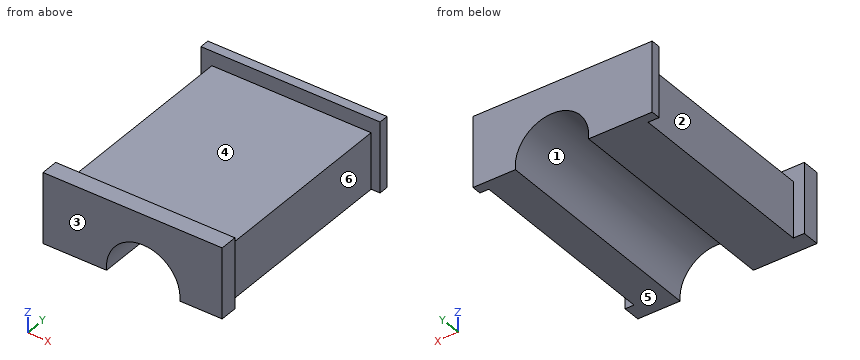
from build123d import *

# Parameters (mm, degrees)
F1_DEPTH = 80
F2_W     = 70.4753454775
F2_H     = 5.0733083159
F3_DEPTH = 64
F4_W     = 3.8940757513
F4_H     = 70.4753454775
F5_DEPTH = 25
F4_W_2   = 3.1526088715
F6_DEPTH = 25


with BuildPart() as f1:
    # F0 (on Front) → F1 (new body)
    with BuildSketch(Plane.XZ):
        with BuildLine():
            Line((-37.5057458878, 24.8617598087), (-37.5057458878, 0))
            Line((-37.5057458878, 0), (-15.074656345, 0))
            ThreePointArc((-15.074656345, 0), (-2.17074994, 14.2445032908), (10.733156465, 0))
            Line((10.733156465, 0), (25.6872158498, 0))
            Line((25.6872158498, 0), (25.6872158498, 24.8617598087))
            Line((25.6872158498, 24.8617598087), (-37.5057458878, 24.8617598087))
        make_face()
    extrude(amount=F1_DEPTH)

    # F2 (on face) → F3 (cut)
    with BuildSketch(Plane(origin=(-37.5057458878, 0, 0), x_dir=(0, -1, 0), z_dir=(-1, 0, 0))):
        with Locations((38.6002035812, 22.3251056507)):
            Rectangle(F2_W, F2_H)
    extrude(amount=-F3_DEPTH, mode=Mode.SUBTRACT)

    # F4 (on face) → F5 (cut)
    with BuildSketch(Plane.XY.offset(19.7884514928)):
        with Locations((-35.5587080121, -38.6002035812)):
            Rectangle(F4_W, F4_H)
    extrude(amount=-F5_DEPTH, mode=Mode.SUBTRACT)

    # F4 (on face) → F6 (cut)
    with BuildSketch(Plane.XY.offset(19.7884514928)):
        with Locations((24.110911414, -38.6002035812)):
            Rectangle(F4_W_2, F4_H)
        with Locations((-35.5587080121, -38.6002035812)):
            Rectangle(F4_W, F4_H)
    extrude(amount=-F6_DEPTH, mode=Mode.SUBTRACT)


solid = f1.part
The listing builds one solid part. Answer for the finished solid, in the listing's coordinates (mm). Face numbers are marked on the shaded views. A direction names the side the tool comes from. Round coordinates to 2 decimals unless told otherwise and drop trailing zeros. Loops run counter-clockwise (first coordinate to the right, second up) from the corner with the lowest first, then second, coordinate; pieces in that order, holes last. Notation, with made-up numbers: M 32,12 L 87,12 A22 ccw 87,47 Z; hole C 75,43.25 d4. An arc over 180 degrees is marked long. Return JSON: item names as keys, results as strings.
Q1. Find section D-D, the plane z = 11.75. Determine the outline of the cut face in (x, y), plus the area to 3 significant figures.
Results list:
{"outline": "M -37.51,-80 L -9.82,-80 L -9.82,0 L -37.51,0 L -37.51,-3.36 L -33.61,-3.36 L -33.61,-73.84 L -37.51,-73.84 Z; M 5.48,-80 L 25.69,-80 L 25.69,-73.84 L 22.53,-73.84 L 22.53,-3.36 L 25.69,-3.36 L 25.69,0 L 5.48,0 Z", "area": "3,340 mm2"}
Q2. Each of these flat-tipped pins is pushed along its axis until it touches: pin 1 Ø1 at (x, y) = (2, -9.5) entering from +Z; pin 2 Ø6 at (y, z) = (-27.5, 10) entering from -X; pin 3 Ø3 at (y, z) = (-35.5, 14) entering from +X. Where does it stop, or does it pass through?
Results list:
{"pin 1": "stops at z = 19.79", "pin 2": "stops at x = -33.61", "pin 3": "stops at x = 22.53"}
Q3. Find the intervals of material crossed by line 1 along Y through (x, z) = (-30, 22); line 2 along X through (y, z) = (-10, 2.5); line 3 along Z through (x, y) = (-16, -25), in increasing order. Write a range as from..to.
Results list:
{"line 1": "y = -80..-73.84, -3.36..0", "line 2": "x = -33.61..-15.08, 10.74..22.53", "line 3": "z = 0..19.79"}
Q4. The mould has two halves that part along X. Classify the marked faces 1, 2 and 3: released by +X, released by -X, zero draft, split by the parting line, or undercut.
Results list:
{"face 1": "undercut", "face 2": "released by -X", "face 3": "zero draft"}
Q5. Find section B-B, the plane x = 13. Determine the outline of the cut face in (y, z), plus the area to 3 significant figures.
Results list:
{"outline": "M -80,0 L 0,0 L 0,24.86 L -3.36,24.86 L -3.36,19.79 L -73.84,19.79 L -73.84,24.86 L -80,24.86 Z", "area": "1,630 mm2"}
Q6. Find section A-A, the plane z = 6.25. Determine the outline of the cut face in (x, y), plus the area to 3 significant figures.
Results list:
{"outline": "M -37.51,-80 L -14.15,-80 L -14.15,0 L -37.51,0 L -37.51,-3.36 L -33.61,-3.36 L -33.61,-73.84 L -37.51,-73.84 Z; M 9.8,-80 L 25.69,-80 L 25.69,-73.84 L 22.53,-73.84 L 22.53,-3.36 L 25.69,-3.36 L 25.69,0 L 9.8,0 Z", "area": "2,640 mm2"}
Q7. Which of the six approach directions +Z, -Z, +X, -X, +Y, -Y give full straight-line access (tool end or side, diameter ignored) to the marked faces 4, 5 and 6?
Results list:
{"face 4": "+Z, +X, -X", "face 5": "-Z, +X, -X, +Y, -Y", "face 6": "+Z, -Z, +X"}
Q8. Find section C-C, the plane y = -65. Determine the outline of the cut face in (x, z).
Results list:
{"outline": "M -33.61,0 L -15.07,0 A12.97 cw long 10.73,0 L 22.53,0 L 22.53,19.79 L -33.61,19.79 Z"}
